Geometry: final body of the model. Coordinates: model frame, mm. Face numbers are marked on the shaded views. A direction names the side the tool comes from. Give positions to 0.01 mm unless a question says otherwise; leave off trailing zeros. Order: outer loops, then holes, each group sorted by start corner. A loop starts at its lowest first (then second) coordinate and runs counter-clockwise, first axis right, second up. Notation, with made-up numbers: (61.25, 0.25) - (79.25, 0.25) arc R15 ccw to (79.25, 12.25) - close; hole circle Ø6 at (-15.5, 71). An arc over 180 degrees is marked (long way). One line per question, with ' | ' between items. Start each with the question number.
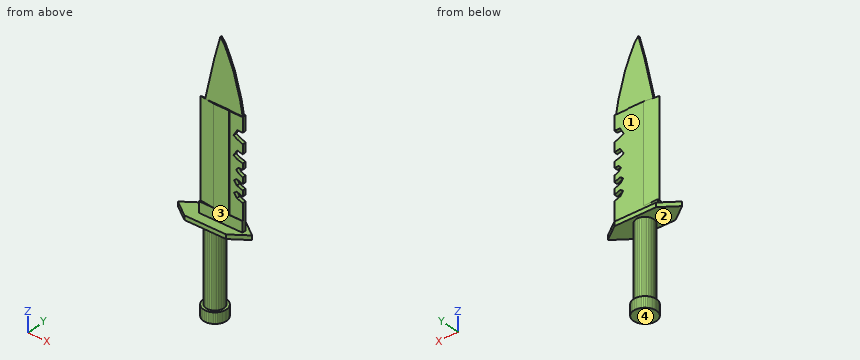
from build123d import *

# Parameters (mm, degrees)
F1_DEPTH  = 12.7
F3_DEPTH  = 88.9
F4_W      = 49.5914556086
F4_H      = 27.8375800699
F5_DEPTH  = 5.08
F7_DEPTH  = 5.08
F8_DEPTH  = 5.08
F9_W      = 51.6053037718
F9_H      = 4.4333104743
F10_DEPTH = 12.7
F11_W     = 18.5319427401
F11_H     = 4.4333104743
F12_DEPTH = 114.3
F14_DEPTH = 114.3
F16_DEPTH = 4.064
F18_DEPTH = 1.016
F19_DEPTH = 1.016


# Not quite as in the source:
# - a length typed as a fraction of an inch, garbled in the dataset ("3 / 203.2 mm" for 3/8 in), is restored


with BuildPart() as f1:
    # F0 (on Top) → F1 (new body)
    with BuildSketch(Plane.XY):
        Polygon((7.6455804064, -11.218967169), (8.9914021538, -10.1722569471), (10.195424118, -8.9651241566), (11.2386581535, -7.6166060026), (12.1046518362, -6.147969422), (12.7797479285, -4.582375691), (13.2532997617, -2.9445151579), (13.5178391405, -1.2602178619), (13.569194121, 0.4439538226), (13.4065548043, 2.1411240902), (13.0324861096, 3.8045275518), (12.4528873238, 5.4079313412), (11.6768990658, 6.9260488228), (10.7167591342, 8.334938377), (9.5876095091, 9.612380974), (8.3072575547, 10.7382305809), (6.8958951862, 11.6947318768), (5.3757804312, 12.4668002649), (3.7708864074, 13.0422597655), (2.1065232524, 13.4120350386), (0.4089389673, 13.5702945071), (-1.2950945296, 13.5145423248), (-2.9787036121, 13.2456577368), (-4.6153367593, 12.7678812137), (-6.1791832887, 12.0887475767), (-7.6455804064, 11.218967169), (-8.9914021538, 10.1722569471), (-10.195424118, 8.9651241566), (-11.2386581535, 7.6166060026), (-12.1046518362, 6.147969422), (-12.7797479285, 4.582375691), (-13.2532997617, 2.9445151579), (-13.5178391405, 1.2602178619), (-13.569194121, -0.4439538226), (-13.4065548043, -2.1411240902), (-13.0324861096, -3.8045275518), (-12.4528873238, -5.4079313412), (-11.6768990658, -6.9260488228), (-10.7167591342, -8.334938377), (-9.5876095091, -9.612380974), (-8.3072575547, -10.7382305809), (-6.8958951862, -11.6947318768), (-5.3757804312, -12.4668002649), (-3.7708864074, -13.0422597655), (-2.1065232524, -13.4120350386), (-0.4089389673, -13.5702945071), (1.2950945296, -13.5145423248), (2.9787036121, -13.2456577368), (4.6153367593, -12.7678812137), (6.1791832887, -12.0887475767), align=None)
    extrude(amount=F1_DEPTH)

    # F2 (on face) → F3 (join)
    with BuildSketch(Plane.XY.offset(12.7)):
        Polygon((2.1904929984, -10.2495944917), (3.7669142259, -9.7807363749), (5.2505815234, -9.0710440681), (6.6049620782, -8.1379925514), (7.796706546, -7.0045566495), (8.7964702228, -5.6986453162), (9.5796356089, -4.2524144224), (10.1269185734, -2.7014749726), (10.4248431933, -1.0840162433), (10.4660735757, 0.5601345635), (10.2495944917, 2.1904929984), (9.7807363749, 3.7669142259), (9.0710440681, 5.2505815234), (8.1379925514, 6.6049620782), (7.0045566495, 7.796706546), (5.6986453162, 8.7964702228), (4.2524144224, 9.5796356089), (2.7014749726, 10.1269185734), (1.0840162433, 10.4248431933), (-0.5601345635, 10.4660735757), (-2.1904929984, 10.2495944917), (-3.7669142259, 9.7807363749), (-5.2505815234, 9.0710440681), (-6.6049620782, 8.1379925514), (-7.796706546, 7.0045566495), (-8.7964702228, 5.6986453162), (-9.5796356089, 4.2524144224), (-10.1269185734, 2.7014749726), (-10.4248431933, 1.0840162433), (-10.4660735757, -0.5601345635), (-10.2495944917, -2.1904929984), (-9.7807363749, -3.7669142259), (-9.0710440681, -5.2505815234), (-8.1379925514, -6.6049620782), (-7.0045566495, -7.796706546), (-5.6986453162, -8.7964702228), (-4.2524144224, -9.5796356089), (-2.7014749726, -10.1269185734), (-1.0840162433, -10.4248431933), (0.5601345635, -10.4660735757), align=None)
    extrude(amount=F3_DEPTH)

    # F4 (on face) → F5 (join)
    with BuildSketch(Plane.XY.offset(101.6)):
        Rectangle(F4_W, F4_H)
    extrude(amount=F5_DEPTH)

    # F6 (on face) → F7 (join)
    with BuildSketch(Plane(origin=(0, 0, 101.6), x_dir=(1, 0, 0), z_dir=(0, 0, -1))):
        Polygon((-44.2462861538, 0), (-24.7957278043, -13.9187900349), (-24.7957278043, 13.9187900349), align=None)
    extrude(amount=-F7_DEPTH)

    # F6 (on face) → F8 (join)
    with BuildSketch(Plane(origin=(0, 0, 101.6), x_dir=(1, 0, 0), z_dir=(0, 0, -1))):
        Polygon((24.7957278043, 13.9187900349), (24.7957278043, -13.9187900349), (44.2214161158, 0), align=None)
    extrude(amount=-F8_DEPTH)

    # F9 (on face) → F10 (join)
    with BuildSketch(Plane.XY.offset(106.68)):
        with Locations((8.7059200741, 0.0440463773)):
            Rectangle(F9_W, F9_H)
    extrude(amount=F10_DEPTH)

    # F11 (on face) → F12 (join)
    with BuildSketch(Plane.XY.offset(119.38)):
        with Locations((9.26597137, 0.0440463773)):
            Rectangle(F11_W, F11_H)
    extrude(amount=F12_DEPTH)

    # F13 (on face) → F14 (join)
    with BuildSketch(Plane.XY.offset(119.38)):
        Polygon((0, -2.1726088598), (0, 2.2607016144), (-17.0967318118, 0), align=None)
    extrude(amount=F14_DEPTH)

    # F15 (on face) → F16 (join)
    with BuildSketch(Plane(origin=(0, 2.2607016144, 0), x_dir=(-1, 0, 0), z_dir=(0, 1, 0))):
        Polygon((-34.50857196, 124.4318857789), (-34.50857196, 119.38), (-18.5319427401, 119.38), (-18.5319427401, 233.0740690231), (-34.50857196, 233.0740690231), (-34.50857196, 216.0275018554), (-27.85702236, 216.0275018554), (-23.4947055578, 208.6254060268), (-27.85702236, 206.0545384884), (-34.50857196, 203.4297866207), (-34.50857196, 192.3147596109), (-27.85702236, 193.8075326945), (-23.4947055578, 186.8935078382), (-27.85702236, 184.1411590576), (-34.50857196, 182.4075117771), (-34.50857196, 175.4231682831), (-29.6370955184, 175.4231682831), (-26.5028076246, 172.5162565708), (-29.6370955184, 169.1368073225), (-34.50857196, 167.0584704934), (-34.50857196, 159.7376912832), (-27.4633802474, 162.3028325299), (-24.0699224556, 159.7376912832), (-27.4633802474, 155.2484430598), (-34.50857196, 152.6833018131), (-34.50857196, 145.9243744612), (-27.4633802474, 148.4895157079), (-24.0699224556, 145.9243744612), (-27.4633802474, 141.4351262377), (-34.50857196, 138.869984991), (-34.50857196, 131.7707747221), align=None)
    extrude(amount=-F16_DEPTH)

    # F17 (on Front) → F18 (join)
    with BuildSketch(Plane.XZ):
        Polygon((-10.8600538224, 233.6585074663), (33.719830215, 233.0019772053), (30.6109376252, 250.2144873142), (27.6256743819, 260.3836655617), (23.0536255985, 277.1858274937), (16.9042795897, 292.2313511372), (11.6809960455, 303.2293915749), (7.1772807278, 309.0918958187), (0, 282.517939806), align=None)
    extrude(amount=F18_DEPTH)

    # F17 (on Front) → F19 (join)
    with BuildSketch(Plane.XZ):
        Polygon((-10.8600538224, 233.6585074663), (33.719830215, 233.0019772053), (30.6109376252, 250.2144873142), (27.6256743819, 260.3836655617), (23.0536255985, 277.1858274937), (16.9042795897, 292.2313511372), (11.6809960455, 303.2293915749), (7.1772807278, 309.0918958187), (0, 282.517939806), align=None)
    extrude(amount=-F19_DEPTH)


solid = f1.part
(1) Cut plane C-C, the plane x = 39. Return the cut outline in (y, z), plus the area to 3 significant figures.
(2) Cut plane B-B, the plane x = -36. Return the cut outline in (y, z).
(3) Cut plane A-A, the plane z = 225. Return the cut outline in (x, y).
(4) Material intervals for line 1 along Z through (x, y) = (9.5, 5.25); line 2 along Y through (x, z) = (10, 261); line 3 along Z through (x, y) = (-12.5, 9), sorted ascending. Write a range as from..to.
(5) Access query for the marked faces 1, 2, 3 and 4. Directions: +Z, -Z, +X, -X, +Y, -Y. A direction counts if a zero-diameter tool reaches every point of the face in a straight line with its end or side. Return the directions, or none.
(6) Contact query for flat-ended pins moving along their axis: P1, Ø2, axis at y = 1, z = 125, coming from the +X side; P2, Ø12, axis at y = 3.5, z = 86.5, coming from the +X side; P3, Ø22.5, axis at x = 2.5, z = 273, coming from the -Y side. Output: stop coordinate, or through.
Results are:
1) outline: (-3.74, 101.6) - (3.74, 101.6) - (3.74, 106.68) - (-3.74, 106.68) - close | area: 38.0 mm2
2) outline: (-5.9, 101.6) - (5.9, 101.6) - (5.9, 106.68) - (-5.9, 106.68) - close
3) outline: (-17.1, 0) - (0, -2.17) - (18.53, -2.17) - (18.53, -1.8) - (34.51, -1.8) - (34.51, 2.26) - (0, 2.26) - close
4) line 1: 0..12.7, 101.6..106.68 | line 2: -1.02..1.02 | line 3: 101.6..106.68
5) face 1: +Z, +X, -X, +Y | face 2: none | face 3: +Z, +X, -X, -Y | face 4: -Z, +X, -X, +Y, -Y
6) P1: x = 34.51 | P2: x = 10.47 | P3: y = -1.02
